```python
from build123d import *

# Parameters (mm, degrees)
EXTRUDE_1_DEPTH              = 2.4
SKETCH_2_R                   = 2.75
EXTRUDE_2_DEPTH              = 3.9
FILLET_1_R                   = 0.7
FILLET_2_R                   = 0.2
HOLE_WIZARD_M3_1_D           = 2.5
HOLE_WIZARD_M3_1_DEPTH       = 7.5
HOLE_WIZARD_M3_1_CSINK_D     = 3.05
HOLE_WIZARD_M3_1_CSINK_ANGLE = 90
HOLE_WIZARD_M3_1_TIP         = 0.751075774


with BuildPart() as part:
    # 草图1 → 凸台-拉伸1 (new body)
    with BuildSketch(Plane(origin=(0, 0, 0), x_dir=(1, 0, 0), z_dir=(0, 1, 0))):
        Polygon((2.75, -1.58771324), (2.75, 1.58771324), (0, 3.175426481), (-2.75, 1.58771324), (-2.75, -1.58771324), (0, -3.175426481), align=None)
    extrude(amount=EXTRUDE_1_DEPTH)

    # 草图2 → 凸台-拉伸2 (add)
    with BuildSketch(Plane.XZ):
        Circle(SKETCH_2_R)
    extrude(amount=-EXTRUDE_2_DEPTH)

    # 圆角1
    fillet_1_edges = [part.edges().sort_by_distance(p)[0] for p in [
        (-2.75, 3.9, 0),
    ]]
    fillet(fillet_1_edges, radius=FILLET_1_R)

    # 圆角2
    fillet_2_edges = [part.edges().sort_by_distance(p)[0] for p in [
        (0, 1.2, 3.175426481),
        (-2.75, 1.2, 1.58771324),
        (-2.75, 1.2, -1.58771324),
        (0, 1.2, -3.175426481),
        (2.75, 1.2, -1.58771324),
        (2.75, 1.2, 1.58771324),
    ]]
    fillet(fillet_2_edges, radius=FILLET_2_R)

    # M3 螺纹孔1
    with Locations(Plane(origin=(0, 0, 0), x_dir=(-1, 0, 0), z_dir=(0, -1, 0))):
        with Locations((0, 0)):
            CounterSinkHole(HOLE_WIZARD_M3_1_D / 2, HOLE_WIZARD_M3_1_CSINK_D / 2, depth=HOLE_WIZARD_M3_1_DEPTH, counter_sink_angle=HOLE_WIZARD_M3_1_CSINK_ANGLE)
            with Locations((0, 0, -(HOLE_WIZARD_M3_1_DEPTH + HOLE_WIZARD_M3_1_TIP / 2))):  # 118° drill point
                Cone(0, HOLE_WIZARD_M3_1_D / 2, HOLE_WIZARD_M3_1_TIP, mode=Mode.SUBTRACT)


solid = part.part
```
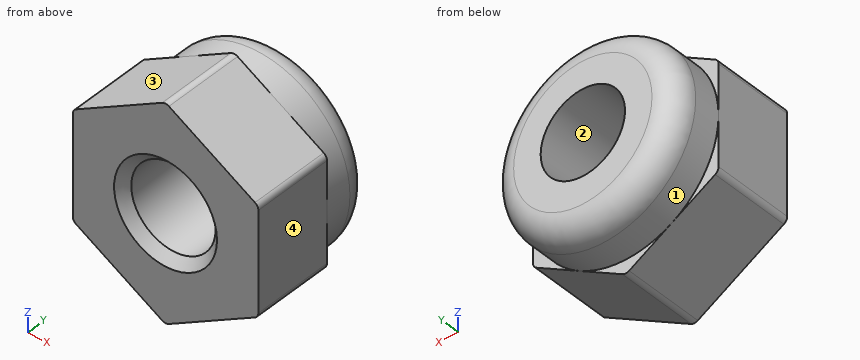
Geometry check sheet. Reference: the model listing, model coordinates, mm. Face numbers are marked on the shaded views. Round coordinates to 2 decimals unless told otherwise and drop trailing zeros. Order: outer loops, then holes, each group sorted by start corner. A loop starts at its lowest first (then second) coordinate and runs counter-clockwise, first axis right, second up. Notation, with made-up numbers: (-39.75, -12.5) - (-14.75, -12.5) arc R18 cw to (-14.75, -0.5) - close; hole circle Ø11 at (-38, 28.25). An arc over 180 degrees is marked (long way). Use a Markdown table: item, result. Add a question column.
(1) Sectioned sample at A-A, the plane y = 1.6. Enter the section's corners in (x, z), and give its area (3 significant figures).
(2) Sectioned sample at C-C, the plane y = 3.3. Enter the section's corners in (x, z), and give its area (3 significant figures).
(3) Sectioned sample at B-B, the plane x = 0. Enter the section's corners in (y, z) (3 decimals), and give its area (3 significant figures).
(4) Depth check by flat-ended pin: pin 1 (3 mm diameter, centred on x = 0, z = 0, fed in from -Y) (3 decimals). Enter the tip coordinate at first touch or a pass-through.
(5) Release check for a two-part mould opening along X. For the marked faces 1, 2, 3 and 4 record: pulls with the +X half, pulls with the -X half, needs draft (parallel to the pull), parting line crosses it, or undercut.
(6) Material ranges on line 1 along Z through (x, y) = (0, 2.3); line 2 along Z through (x, y) = (0, 2.9); line 3 along X through (y, z) = (0.75, -0.75), recorded low to high. Write a range as [from, to].
Answers below:
| question | item | result |
|---|---|---|
| 1 | outline | (-2.75, -1.47) arc R0.2 ccw to (-2.65, -1.65) - (-0.1, -3.12) arc R0.2 ccw to (0.1, -3.12) - (2.65, -1.65) arc R0.2 ccw to (2.75, -1.47) - (2.75, 1.47) arc R0.2 ccw to (2.65, 1.65) - (0.1, 3.12) arc R0.2 ccw to (-0.1, 3.12) - (-2.65, 1.65) arc R0.2 ccw to (-2.75, 1.47) - close; hole circle Ø2.5 at (0, 0) |
| 1 | area | 21.3 mm² |
| 2 | outline | circle Ø5.49 at (0, 0); hole circle Ø2.5 at (0, 0) |
| 2 | area | 18.7 mm² |
| 3 | outline | (0, -3.144) - (2.4, -3.144) - (2.4, -2.75) - (3.2, -2.75) arc R0.7 ccw to (3.9, -2.05) - (3.9, -1.25) - (0.275, -1.25) - (0, -1.525) - close; (0, 1.525) - (0.275, 1.25) - (3.9, 1.25) - (3.9, 2.05) arc R0.7 ccw to (3.2, 2.75) - (2.4, 2.75) - (2.4, 3.144) - (0, 3.144) - close |
| 3 | area | 13.3 mm² |
| 4 | pin 1 | y = 0.025 |
| 5 | face 1 | parting line crosses it |
| 5 | face 2 | undercut |
| 5 | face 3 | pulls with the -X half |
| 5 | face 4 | pulls with the +X half |
| 6 | line 1 | [-3.14, -1.25], [1.25, 3.14] |
| 6 | line 2 | [-2.75, -1.25], [1.25, 2.75] |
| 6 | line 3 | [-2.75, -1], [1, 2.75] |
